Here's how the part is built. I have some questions about the finished solid (model axes, mm). A direction names the side the tool comes from. Coordinates: 2 decimals unless noted, no trailing zeros. Loops run counter-clockwise (first coordinate to the right, second up) from the corner with the lowest first, then second, coordinate; pieces in that order, holes last. Notation, with made-up numbers: M -24.75,57 L 19.25,57 A19 ccw 19.25,66 Z; hole C -3,43 d4. An arc over 180 degrees is marked long. Use CSV: the item, a comma, the result in double quotes. Start each with the question number.
Q1. If we section it at C-C (y = -6.5): Please give me the cut outline in (x, z).
Q2. If we section it at A-A (z = 0): Please give me the cut outline in (x, y).
Q3. Which directions (+Z, -Z, +X, -X, +Y, -Y) give clear straight access to the entire face, cutting with the end or side of a thin tool? Please do faces 1 (the flat face through (0.1, -15, 3.2)), 2 (the flat face through (0, 0, 0)).
Q4. If we section it at D-D (y = -60.5): Please give me the cut outline in (x, z), and give its area (3 significant figures).
Q5. For pin 1 Ø1.5 at (x, z) = (-2, 5.5) entering from -Y; pin 2 Ø3 at (x, y) = (4, -58.5) entering from +Z; pin 3 Ø1 at (x, z) = (1, 0) entering from -Y, each with a flat end and sliding along its axis, tell me the tip position at first contact or that it passes through.
Q6. Please list where these lines run through material, in increasing order: probe 1 along X at (y, z) = (-58, 0); probe 2 along Y at (x, z) = (0, 5); probe 3 along X at (y, z) = (-62, 1.5). Write a range as [from, to].
Q7. If we section it at B-B (x = 0): Please give me the cut outline in (y, z), and give its area (3 significant figures).
Q8. If we mould it in two halves opening along X, with no side actions, what happens to faces 3 (the flat face through (2, -65, 0)), 4 (the cylindrical face through (-1, -59.08, -1.31)), 5 (the cylindrical face through (0.33, -7.395, -7.493)), 6 (the flat face through (0, -53, 0))? For each: +X half, -X half, draft (parallel to the pull), parting line (faces both ways), or undercut.
from build123d import *

# Parameters (mm, degrees)
SKETCH1_R           = 7.5
BOSS_EXTRUDE1_DEPTH = 15
SKETCH3_R           = 2.9
BOSS_EXTRUDE3_DEPTH = 50
SKETCH4_R           = 1.65
CUT_EXTRUDE1_DEPTH  = 12


with BuildPart() as part:
    # Sketch1 → Boss-Extrude1 (new body)
    with BuildSketch(Plane(origin=(0, 0, 0), x_dir=(1, 0, 0), z_dir=(0, 1, 0))):
        with Locations(Location((0, 0, 0), (0, 0, 270))):
            Circle(SKETCH1_R)
    extrude(amount=-BOSS_EXTRUDE1_DEPTH)

    # Sketch3 → Boss-Extrude3 (add)
    with BuildSketch(Plane.XZ.offset(15)):
        with Locations(Location((0, 0, 0), (0, 0, 90))):
            Circle(SKETCH3_R)
    extrude(amount=BOSS_EXTRUDE3_DEPTH)

    # Sketch4 → Cut-Extrude1 (cut)
    with BuildSketch(Plane(origin=(0, -65, 0), x_dir=(1, 0, 0), z_dir=(0, 1, 0))):
        with Locations(Location((0, 0, 0), (0, 0, 270))):
            Circle(SKETCH4_R)
    extrude(amount=CUT_EXTRUDE1_DEPTH, mode=Mode.SUBTRACT)


solid = part.part
Results below:
1,outline,"C 0,0 d15"
2,outline,"M -7.5,-15 L -2.9,-15 L -2.9,-65 L -1.65,-65 L -1.65,-53 L 1.65,-53 L 1.65,-65 L 2.9,-65 L 2.9,-15 L 7.5,-15 L 7.5,0 L -7.5,0 Z"
3,face 1,"-Y"
3,face 2,"+Z, -Z, +X, -X, +Y"
4,outline,"C 0,0 d5.8; hole C 0,0 d3.3"
4,area,"17.9 mm^2"
5,pin 1,"y = -15"
5,pin 2,"z = 1.47"
5,pin 3,"y = -53"
6,probe 1,"[-2.9, -1.65], [1.65, 2.9]"
6,probe 2,"[-15, 0]"
6,probe 3,"[-2.48, -0.69], [0.69, 2.48]"
7,outline,"M -65,-2.9 L -15,-2.9 L -15,-7.5 L 0,-7.5 L 0,7.5 L -15,7.5 L -15,2.9 L -65,2.9 L -65,1.65 L -53,1.65 L -53,-1.65 L -65,-1.65 Z"
7,area,"475 mm^2"
8,face 3,"draft"
8,face 4,"undercut"
8,face 5,"parting line"
8,face 6,"undercut"
